Source: CAD feature listing. Evaluate the final solid. Frame: model axes, mm. A direction names the side the tool comes from. Round coordinates to 2 decimals unless told otherwise and drop trailing zeros. Order: outer loops, then holes, each group sorted by start corner. A loop starts at its lowest first (then second) coordinate and runs counter-clockwise, first axis right, second up. Notation, with made-up numbers: (13, 22.5) - (61, 22.5) arc R19 cw to (61, 43.5) - close; hole circle Ø1 at (16, 71). An arc over 180 degrees is marked (long way). Put each result on its own line as item: value. Start each with the question number.
1) Section A-A on z = 0. Output: boundary loops of the cut face in (x, y).
2) Section B-B on x = 0. Output: boundary loops of the cut face in (y, z).
3) Access query for faces 4 (the face through (-22.9, 3.9, -39.2)), 5 (the face through (0, 4, -55)). Directions: +Z, -Z, +X, -X, +Y, -Y. A direction counts if a zero-diameter tool reaches every point of the face in a straight line with its end or side. Return the directions, or none.
4) Line query: probe 1 along Z at (x, y) = (0, 5); probe 2 along X at (y, z) = (4, 0); probe 3 along Z at (x, y) = (19, 2). Output: solid intervals per line, ascending. Write a range as [from, to].
5) Mould query, pull axis X, two halves, no side actions, for faces 1 (the face through (22.9, 3.9, 39.2)), 2 (the face through (38.5, 4.1, -53.5)), 3 (the face through (0, 4, 55)). Classes: +X half, -X half, draft (parallel to the pull), parting line (faces both ways), or undercut.
6) Contact query for a flat-ended pin moving along its axis: P1, Ø5, axis at x = -26, z = 6.5, coming from the -Y side. Output: stop coordinate, or through.
7) Section C-C on y = 6.25. Output: boundary loops of the cut face in (x, z), then the cut area to 3 significant figures.
8) Section D-D on x = 31.5. Output: boundary loops of the cut face in (y, z).
Autodesk Fusion 360 part; units mm, degrees
sketch "Sketch1" plane through (0, 0, 0) normal (0, 1, 0) x (1, 0, 0)
  line L0 (22.9749, 31.6447) -> (-22.9749, 31.6447) construction
  line L1 (-22.9749, 31.6447) -> (-22.9749, -31.6447) construction
  line L2 (-22.9749, -31.6447) -> (22.9749, -31.6447) construction
  line L3 (22.9749, -31.6447) -> (22.9749, 31.6447) construction
  line L4 (22.9749, 31.6447) -> (-22.9749, -31.6447) construction
  line L5 (-22.9749, 31.6447) -> (22.9749, -31.6447) construction
  line L6 (30.0251, 41.3553) -> (-30.0251, 41.3553) construction
  line L7 (-30.0251, 41.3553) -> (-30.0251, -41.3553) construction
  line L8 (-30.0251, -41.3553) -> (30.0251, -41.3553) construction
  line L9 (30.0251, -41.3553) -> (30.0251, 41.3553) construction
  line L10 (30.0251, 41.3553) -> (-30.0251, -41.3553) construction
  line L11 (-30.0251, 41.3553) -> (30.0251, -41.3553) construction
  line L12 (26.6164, 29.0009) -> (33.6665, 38.7115)
  arc A0 (33.6665, 38.7115) -> (26.3836, 43.9991) centre (30.0251, 41.3553) ccw
  line L13 (26.3836, 43.9991) -> (19.3335, 34.2885)
  arc A1 (19.3335, 34.2885) -> (26.6164, 29.0009) centre (22.9749, 31.6447) ccw
  line L14 (22.9749, 31.6447) -> (30.0251, 41.3553) construction
  line L15 (0, 0) -> (0, 52.4802) construction
  line L16 (0, 0) -> (-40, 0) construction
  arc A2 (-26.3836, 43.9991) -> (-33.6665, 38.7115) centre (-30.0251, 41.3553) ccw
  line L17 (-26.6164, 29.0009) -> (-33.6665, 38.7115)
  arc A3 (-26.6164, 29.0009) -> (-19.3335, 34.2885) centre (-22.9749, 31.6447) ccw
  line L18 (-26.3836, 43.9991) -> (-19.3335, 34.2885)
  arc A4 (-33.6665, -38.7115) -> (-26.3836, -43.9991) centre (-30.0251, -41.3553) ccw
  line L19 (-26.3836, -43.9991) -> (-19.3335, -34.2885)
  line L20 (-26.6164, -29.0009) -> (-33.6665, -38.7115)
  arc A5 (-19.3335, -34.2885) -> (-26.6164, -29.0009) centre (-22.9749, -31.6447) ccw
  line L21 (26.3836, -43.9991) -> (19.3335, -34.2885)
  arc A6 (26.3836, -43.9991) -> (33.6665, -38.7115) centre (30.0251, -41.3553) ccw
  line L22 (26.6164, -29.0009) -> (33.6665, -38.7115)
  arc A7 (26.6164, -29.0009) -> (19.3335, -34.2885) centre (22.9749, -31.6447) ccw
  line L23 (39.9315, 55) -> (-39.9315, 55)
  line L24 (-39.9315, 55) -> (-39.9315, -55)
  line L25 (-39.9315, -55) -> (39.9315, -55)
  line L26 (39.9315, -55) -> (39.9315, 55)
  line L27 (39.9315, 55) -> (-39.9315, -55) construction
  line L28 (-39.9315, 55) -> (39.9315, -55) construction
  circle A8 centre (0, 0) radius 16.5
  line L29 (26.5, 36.5) -> (24.038, 38.2875) construction
  point P0 (26.5, 36.5)
  point P1 (-26.5, 36.5)
  point P2 (26.5, -36.5)
  point P3 (-26.5, -36.5)
  dimension "d1" = 4.5
  dimension "d2" = 12
  dimension "d5" = 110
  dimension "d9" = 33
  dimension "d11" = 73
  dimension "d13" = 53
extrude "Extrude1" add sketch "Sketch1" along normal blind 8
fillet "Fillet1" radius 5 4 edges at (39.9315, 4, -55) (-39.9315, 4, 55) (39.9315, 4, 55) (-39.9315, 4, -55)
equation "d1 = ( 9 / 2 ) * 1 mm"
Answer sheet:
1. outline: (-39.93, 0) - (-16.5, 0) - (-16.5, 8) - (-39.93, 8) - close; (16.5, 0) - (39.93, 0) - (39.93, 8) - (16.5, 8) - close
2. outline: (0, -55) - (8, -55) - (8, -16.5) - (0, -16.5) - close; (0, 16.5) - (8, 16.5) - (8, 55) - (0, 55) - close
3. face 4: +Y, -Y
3. face 5: -Z, +X, -X, +Y, -Y
4. probe 1: [-55, -16.5], [16.5, 55]
4. probe 2: [-39.93, -16.5], [16.5, 39.93]
4. probe 3: [-55, -33.75], [-29.54, 29.54], [33.75, 55]
5. face 1: undercut
5. face 2: +X half
5. face 3: draft
6. P1: y = 0
7. outline: (-39.93, -50) arc R5 ccw to (-34.93, -55) - (34.93, -55) arc R5 ccw to (39.93, -50) - (39.93, 50) arc R5 ccw to (34.93, 55) - (-34.93, 55) arc R5 ccw to (-39.93, 50) - close; hole (-33.67, -38.71) arc R4.5 ccw to (-26.38, -44) - (-19.33, -34.29) arc R4.5 ccw to (-26.62, -29) - close; hole (-33.67, 38.71) - (-26.62, 29) arc R4.5 ccw to (-19.33, 34.29) - (-26.38, 44) arc R4.5 ccw to start; hole circle Ø33 at (0, 0); hole (19.33, -34.29) - (26.38, -44) arc R4.5 ccw to (33.67, -38.71) - (26.62, -29) arc R4.5 ccw to start; hole (19.33, 34.29) arc R4.5 ccw to (26.62, 29) - (33.67, 38.71) arc R4.5 ccw to (26.38, 44) - close
7. area: 7,220 mm^2
8. outline: (0, -55) - (8, -55) - (8, -45.61) - (0, -45.61) - close; (0, -35.73) - (8, -35.73) - (8, 35.73) - (0, 35.73) - close; (0, 45.61) - (8, 45.61) - (8, 55) - (0, 55) - close
